Design review of the part built by this model. Coordinates are the model's own, in mm. A direction names the side the tool comes from. Round coordinates to 2 decimals unless told otherwise and drop trailing zeros. Loops run counter-clockwise (first coordinate to the right, second up) from the corner with the lowest first, then second, coordinate; pieces in that order, holes last. Notation, with made-up numbers: (76, 47) - (119, 47) arc R27 ccw to (119, 63) - close; hole circle Ø8 at (13, 35.5). An arc over 180 degrees is marked (long way). Return JSON: item names as keys, results as strings. Group by question number.
(1) Wall thickness on L1, parallel to Y at x = 0, z = 1 (3 decimals); L2, parallel to Y at x = -10, z = 1.65; L3, parallel to X at y = 3.75, z = 0.45: over which ranges is each line inside the solid? List them lowest first. Write a range as [from, to].
(2) We need section B-B, the plane x = 0. Write out the cut boundary in (y, z) (3 decimals).
(3) We need section C-C, the plane y = 4.5. Write out the cut boundary in (x, z).
(4) For faces 1 (the flat face through (-26, 0, 1)), 2 (the flat face through (-40, -2.896, 1)), 3 (the flat face through (-20, -2, 2.464)), list the 3-axis set-ups (+Z, -Z, +X, -X, +Y, -Y) from which the entire face can be reached by the end or side of a thin tool; tool diameter is ignored.
(5) Clearance check with flat-ended pins moving along their axes: pin 1 (5 mm diameter, centred on x = 0, y = 0, fed in from -Z); pin 2 (5 mm diameter, centred on x = 1.5, y = 4, fed in from -Z); pin 3 (1.2 mm diameter, centred on x = -39.5, z = 1.5, fed in from -Y); pin 4 (0.7 mm diameter, centred on x = -31, z = 0.5, fed in from +Y). State where each tip first meets the part, or that it passes through.
(6) We need section A-A, the plane z = 1.9. Write out the cut boundary in (x, y) (3 decimals).
(7) The part is to be moulded in two halves that separate along X. For faces 4 (the flat face through (-45.11, -4, 1)), 5 (the flat face through (-28.651, -4, 1)), 6 (the flat face through (-32.004, -4, 1)), 7 (the flat face through (-43, -7.772, 1)), say which applies: pulls with the +X half, pulls with the -X half, needs draft (parallel to the pull), parting line crosses it, or undercut.
from build123d import *

# Parameters (mm, degrees)
F1_DEPTH = 2.46395
F2_D     = 6.35


with BuildPart() as f1:
    # F0 (on Top) → F1 (new body)
    with BuildSketch(Plane.XY):
        with BuildLine():
            ThreePointArc((-6.05011, -2.8956), (1.484625, -6.540965), (6.707334, 0))
            ThreePointArc((6.707334, 0), (0, 6.707334), (-6.707334, 0))
            ThreePointArc((-6.707334, 0), (-6.540965, -1.484625), (-6.05011, -2.8956))
        make_face()
        with BuildLine():
            ThreePointArc((-6.05011, -2.8956), (-6.540965, -1.484625), (-6.707334, 0))
            Line((-6.707334, 0), (-45.110401, 0))
            Line((-45.110401, 0), (-45.110401, -7.772401))
            Line((-45.110401, -7.772401), (-41.757599, -7.772401))
            Line((-41.757599, -7.772401), (-41.757599, -2.8956))
            Line((-41.757599, -2.8956), (-38.4048, -2.8956))
            Line((-38.4048, -2.8956), (-38.4048, -6.2484))
            Line((-38.4048, -6.2484), (-35.052001, -6.2484))
            Line((-35.052001, -6.2484), (-35.052001, -2.8956))
            Line((-35.052001, -2.8956), (-32.003999, -2.8956))
            Line((-32.003999, -2.8956), (-32.003999, -5.334001))
            Line((-32.003999, -5.334001), (-28.651198, -5.334001))
            Line((-28.651198, -5.334001), (-28.651198, -2.8956))
            Line((-28.651198, -2.8956), (-6.05011, -2.8956))
        make_face()
    extrude(amount=F1_DEPTH)

    # F2 (through all)
    with Locations(Plane(origin=(0, 0, 0), x_dir=(1, 0, 0), z_dir=(0, 0, -1))):
        with Locations((0, 0)):
            Hole(F2_D / 2)


solid = f1.part
Solutions:
{
 "1": {"L1": "[-6.707, -3.175], [3.175, 6.707]", "L2": "[-2.9, 0]", "L3": "[-5.56, 5.56]"},
 "2": {"outline": "(-6.707, 0) - (-3.175, 0) - (-3.175, 2.464) - (-6.707, 2.464) - close; (3.175, 0) - (6.707, 0) - (6.707, 2.464) - (3.175, 2.464) - close"},
 "3": {"outline": "(-4.97, 0) - (4.97, 0) - (4.97, 2.46) - (-4.97, 2.46) - close"},
 "4": {"face 1": "+Z, -Z, -X, +Y", "face 2": "+Z, -Z, -Y", "face 3": "+Z, +X, -X, +Y, -Y"},
 "5": {"pin 1": "through", "pin 2": "z = 0", "pin 3": "y = -2.9", "pin 4": "y = 0"},
 "6": {"outline": "(-45.11, -7.772) - (-41.758, -7.772) - (-41.758, -2.896) - (-38.405, -2.896) - (-38.405, -6.248) - (-35.052, -6.248) - (-35.052, -2.896) - (-32.004, -2.896) - (-32.004, -5.334) - (-28.651, -5.334) - (-28.651, -2.896) - (-6.05, -2.896) arc R6.707 ccw (long way) to (-6.707, 0) - (-45.11, 0) - close; hole circle Ø6.35 at (0, 0)"},
 "7": {"face 4": "pulls with the -X half", "face 5": "undercut", "face 6": "undercut", "face 7": "needs draft"}
}
